from build123d import *

# Parameters (mm, degrees)
BOSS_EXTRUDE1_DEPTH      = 1.5
SKETCH1_4_W              = 11
SKETCH1_4_H              = 2
BOSS_EXTRUDE2_DEPTH      = 1
BOSS_EXTRUDE3_DEPTH      = 0.5
BOSS_EXTRUDE3_DEPTH_BACK = 2.5
CUT_EXTRUDE1_DEPTH       = 2.5
CUT_EXTRUDE2_START       = -2
CUT_EXTRUDE2_DEPTH       = 2.5
CUT_EXTRUDE3_DEPTH       = 10
CUT_EXTRUDE4_START       = -0.993883735
CUT_EXTRUDE4_OUTLINE_W   = 14
CUT_EXTRUDE4_OUTLINE_H   = 2
CUT_EXTRUDE4_DEPTH       = 0.993883735
CUT_EXTRUDE5_DEPTH       = 6
CUT_EXTRUDE6_DEPTH       = 6


# Read off the part's stored shape, not the designer's step: Cut-Extrude4
with BuildPart() as part:
    # Sketch1 → Boss-Extrude1 (new, symmetric)
    with BuildSketch(Plane.XY):
        Polygon((-28.5, -6), (-39.5, -6), (-39.5, -9), (-42, -11.5), (-42, -20.5), (-36, -20.5), (-24.008925726, -8.508925726), (-21.5, -6), align=None)
    extrude(amount=BOSS_EXTRUDE1_DEPTH, both=True)

    # Sketch1_4 → Boss-Extrude2 (add, symmetric)
    with BuildSketch(Plane.XY):
        with Locations((-34, -5)):
            Rectangle(SKETCH1_4_W, SKETCH1_4_H)
    extrude(amount=BOSS_EXTRUDE2_DEPTH, both=True)

    # Sketch2 → Boss-Extrude3 (add, two sides: drawn at the far end of the back side and taken through both)
    with BuildSketch(Plane(origin=(0, 0, -1), x_dir=(-1, 0, 0), z_dir=(0, 0, -1)).offset(-BOSS_EXTRUDE3_DEPTH_BACK)):
        Polygon((21.5, -6), (28.5, -6), (20.625, -5.125), align=None)
    extrude(amount=BOSS_EXTRUDE3_DEPTH + BOSS_EXTRUDE3_DEPTH_BACK)

    # Sketch2_3 → Cut-Extrude1 (cut)
    with BuildSketch(Plane(origin=(0, 0, -1), x_dir=(-1, 0, 0), z_dir=(0, 0, -1))):
        Polygon((39.5, -6), (39.5, -7.222222222), (28.5, -6), align=None)
    extrude(amount=CUT_EXTRUDE1_DEPTH, mode=Mode.SUBTRACT)

    # Sketch2_4 → Cut-Extrude2 (cut)
    with BuildSketch(Plane(origin=(0, 0, -1), x_dir=(-1, 0, 0), z_dir=(0, 0, -1)).offset(CUT_EXTRUDE2_START)):
        Polygon((39.5, -6), (39.5, -7.222222222), (28.5, -6), align=None)
    extrude(amount=-CUT_EXTRUDE2_DEPTH, mode=Mode.SUBTRACT)

    # Sketch3 → Cut-Extrude3 (cut)
    with BuildSketch(Plane(origin=(0, 0, -1), x_dir=(-1, 0, 0), z_dir=(0, 0, -1))):
        Polygon((28.5, -4), (39.5, -5.222222222), (39.5, -4), align=None)
    extrude(amount=-CUT_EXTRUDE3_DEPTH, mode=Mode.SUBTRACT)

    # Cut-Extrude4 outline → Cut-Extrude4 (cut)
    with BuildSketch(Plane(origin=(0.091463415, -0.823170732, 0), x_dir=(0.993883734673619, 0.11043152607484619, 0), z_dir=(-0.11043152607484619, 0.993883734673619, 0)).offset(CUT_EXTRUDE4_START)):
        with Locations((-34, 0)):
            Rectangle(CUT_EXTRUDE4_OUTLINE_W, CUT_EXTRUDE4_OUTLINE_H)
    extrude(amount=CUT_EXTRUDE4_DEPTH, mode=Mode.SUBTRACT)

    # Sketch6 → Cut-Extrude5 (cut)
    with BuildSketch(Plane(origin=(0, 0, -1.5), x_dir=(-1, 0, 0), z_dir=(0, 0, -1))):
        Polygon((22.46223447, -5.329137163), (22.29892474, -6.79892474), (20.531436433, -7.019526438), (20.056691247, -4.979132235), (21.915268146, -4.302367821), align=None)
    extrude(amount=-CUT_EXTRUDE5_DEPTH, mode=Mode.SUBTRACT)

    # Sketch7 → Cut-Extrude6 (cut)
    with BuildSketch(Plane(origin=(0, 0, -1.5), x_dir=(-1, 0, 0), z_dir=(0, 0, -1))):
        Polygon((22.29892474, -6.79892474), (36, -20.5), (23.926432251, -5.491825806), (22.46223447, -5.329137163), align=None)
    extrude(amount=-CUT_EXTRUDE6_DEPTH, mode=Mode.SUBTRACT)


solid = part.part
The listing builds one solid part. Answer for the finished solid, in the listing's coordinates (mm). A direction names the side the tool comes from. Give positions to 0.01 mm unless a question says otherwise; leave off trailing zeros. Order: outer loops, then holes, each group sorted by start corner. A loop starts at its lowest first (then second) coordinate and runs counter-clockwise, first axis right, second up. Notation, with made-up numbers: (14.25, -17) - (28.25, -17) arc R19 cw to (28.25, 14) - close; hole circle Ø10 at (49.5, 2). An arc over 180 degrees is marked (long way). One line per item, written item: value. Start each with the question number.
1) The mould has two halves that part along X. Classify faces 1 (the face through (-34, -6, -1)), 2 (the face through (-28.5, -5.5, 0)), 3 (the face through (-34.08, -5.62, -0.01)): released by +X, released by -X, zero draft, split by the parting line, or undercut.
2) A cutting plane is placed at D-D on y = -11. Give the vertices of the cut face in (x, z).
3) Find the intervals of material crossed by L1, parallel to X at y = -14, z = 1.1; L2, parallel to X at y = -7.75, z = -1.3; L3, parallel to Y at x = -36.25, z = -0.8, in increasing order.
4) Given pin 1 Ø0.8 at (y, z) = (-7.5, 0.5) entering from -X; pin 2 Ø0.7 at (x, y) = (-35.5, -6) entering from -Z, each flat-ended and moving along its own axis, determine where each tip first touches the part or whether it passes through.
5) A cutting plane is placed at B-B on z = 0. Give the vertices of the cut face in (x, y).
6) A tool of negligible diameter and unlimited length cuts with its end or side. For faces 4 (the face through (-35, -13, -1.5)), 5 (the face through (-39.5, -8, 0)), 6 (the face through (-34, -6, 1)), from which of +Z, -Z, +X, -X, +Y, -Y can it reach the whole face along a straight path? Write none if from no direction.
7) A cutting plane is placed at A-A on y = -5.75. Give the vertices of the cut face in (x, z).
8) A cutting plane is placed at C-C on x = -39. Give the vertices of the cut face in (y, z), then the cut area to 3 significant figures.
Answer sheet:
1. face 1: zero draft
1. face 2: undercut
1. face 3: released by -X
2. outline: (-41.5, -1.5) - (-28.36, -1.5) - (-28.36, 1.5) - (-41.5, 1.5) - close
3. L1: x = -42 to -30.77
3. L2: x = -39.5 to -25.74
3. L3: y = -20.5 to -5.86
4. pin 1: stops at x = -39.5
4. pin 2: stops at z = -1
5. outline: (-42, -20.5) - (-36, -20.5) - (-23.93, -5.49) - (-28.5, -6) - (-28.5, -5) - (-39.5, -6.22) - (-39.5, -9) - (-42, -11.5) - close
6. face 4: -Z, +X, -X, +Y, -Y
6. face 5: +Z, -Z, -X, +Y
6. face 6: +Z, -X, +Y
7. outline: (-35.25, -1) - (-28.5, -1) - (-28.5, 1) - (-35.25, 1) - close; (-26.25, -1.5) - (-24.13, -1.5) - (-24.13, 1.5) - (-26.25, 1.5) - close
8. outline: (-20.5, -1.5) - (-7.17, -1.5) - (-7.17, -1) - (-6.17, -1) - (-6.17, 1) - (-7.17, 1) - (-7.17, 1.5) - (-20.5, 1.5) - close
8. area: 42.0 mm2
